Can you work these out from the model? Positions are in its coordinate system, mm. Face numbers are marked on the shaded views. Coordinates: 2 decimals unless noted, no trailing zeros. Loops run counter-clockwise (first coordinate to the right, second up) from the corner with the lowest first, then second, coordinate; pieces in that order, holes last.
```python
from build123d import *

# Parameters (mm, degrees)
F0_R     = 8.001
F0_R_2   = 1.744437
F1_DEPTH = 1.5748


with BuildPart() as f1:
    # F0 (on Top) → F1 (new body)
    with BuildSketch(Plane.XY):
        with BuildLine():
            ThreePointArc((2.452167, -12.461014), (9.808989, -8.06683), (12.7, 0))
            ThreePointArc((12.7, 0), (-9.808989, 8.06683), (2.452167, -12.461014))
        make_face()
        Circle(F0_R, mode=Mode.SUBTRACT)
        with BuildLine():
            Line((12.7, -18.100876), (12.7, 0))
            ThreePointArc((12.7, 0), (9.808989, -8.06683), (2.452167, -12.461014))
            Line((2.452167, -12.461014), (3.733975, -18.974695))
            ThreePointArc((3.733975, -18.974695), (8.613387, -22.605128), (12.7, -18.100876))
        make_face()
        with Locations((8.174407, -18.100876)):
            Circle(F0_R_2, mode=Mode.SUBTRACT)
    extrude(amount=F1_DEPTH)


solid = f1.part
```
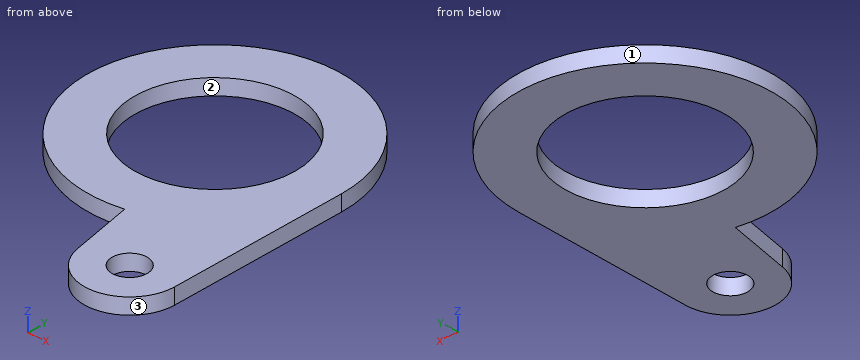
Item 1: I need wall thicknesses on line 1 along Y through (x, z) = (-0.25, 0.85); line 2 along X through (y, z) = (-2.5, 0.45); line 3 along Y through (x, z) = (4.5, 1.05). Which ranges of each line are inside material? Lowest first, please.
Results are:
line 1: y = -12.7 to -8, 8 to 12.7
line 2: x = -12.45 to -7.6, 7.6 to 12.7
line 3: y = -20.74 to -6.62, 6.62 to 11.88
Item 2: Suppose I cut it at A-A, the plane x = 0. Please give me the cut outline in (y, z).
Results are:
outline: (-12.7, 0) - (-8, 0) - (-8, 1.57) - (-12.7, 1.57) - close; (8, 0) - (12.7, 0) - (12.7, 1.57) - (8, 1.57) - close
Item 3: Suppose I cut it at D-D, the plane z = 1.25. Please give me the cut outline in (x, y), plus the area to 3 significant figures.
Results are:
outline: (2.45, -12.46) - (3.73, -18.97) arc R4.53 ccw to (12.7, -18.1) - (12.7, 0) arc R12.7 ccw (long way) to start; hole circle Ø16 at (0, 0); hole circle Ø3.49 at (8.17, -18.1)
area: 415 mm2
Item 4: Suppose I cut it at C-C, the plane x = 7.5. Please give me the cut outline in (y, z), plus the area to 3 significant figures.
Results are:
outline: (-22.58, 0) - (-19.71, 0) - (-19.71, 1.57) - (-22.58, 1.57) - close; (-16.49, 0) - (-2.79, 0) - (-2.79, 1.57) - (-16.49, 1.57) - close; (2.79, 0) - (10.25, 0) - (10.25, 1.57) - (2.79, 1.57) - close
area: 37.8 mm2
Item 5: Suppose I cut it at B-B, the plane y = 0.5. Please give me the cut outline in (x, z), plus the area to 3 significant figures.
Results are:
outline: (-12.69, 0) - (-7.99, 0) - (-7.99, 1.57) - (-12.69, 1.57) - close; (7.99, 0) - (12.69, 0) - (12.69, 1.57) - (7.99, 1.57) - close
area: 14.8 mm2
Item 6: We'd pull the mould along Y, two halves only. Please class the marked faces 1, 2 and 3: +Y half, -Y half, draft (parallel to the pull), parting line (faces both ways), or undercut.
Results are:
face 1: parting line
face 2: undercut
face 3: -Y half
